Could you check a few things on this model? Use its own coordinates, in mm. A direction names the side the tool comes from. Coordinates: 2 decimals unless noted, no trailing zeros. Write each loop counter-clockwise with the first axis right and the second up, starting at its lowest first coordinate (ties: lowest second). Pieces come first, ordered by that corner, then holes.
Item 1: I want a section at B-B on z = 1.55. Please give me the cut outline in (x, y) (3 decimals).
Item 2: If I drill on probe 1 along Y at (x, z) = (9, 2.1) (3 decimals); probe 2 along X at (y, z) = (6.75, 0.6); probe 3 along X at (y, z) = (7.75, 0.65), over which ranges is the centre line in solid material (lowest first)?
Item 3: I want a section at A-A on x = 9.5. Please give me the cut outline in (y, z) (3 decimals), then the cut area to 3 significant figures.
Item 4: Thinking about a two-plate mould opening in X: for faces 3 (the flat face through (21, 6, 2.54)), 4 (the flat face through (34.29, 6, 1)), 5 (the cylindrical face through (3.176, 6.42, 1.288)), 6 (the flat face through (9, 3.175, 1)), which applies, +X half, -X half, draft (parallel to the pull), parting line (faces both ways), or undercut?
Item 5: I want a section at D-D on x = 27. Please give me the cut outline in (y, z), then the cut area to 3 significant figures.
Item 6: For P1, Ø1, axis at y = 4, z = 1, coming from the -X side, with a flat end and sliding along its axis, tell me the tip position at first contact or that it passes through.
Item 7: Which directions (+Z, -Z, +X, -X, +Y, -Y) give clear straight access to the entire face, cutting with the end or side of a thin tool? Please do faces 1 (the flat face through (21, 6, 0)), 2 (the cylindrical face through (15.874, 6.28, 1.288)).
Item 8: I want a section at C-C on y = 6. Please give me the cut outline in (x, z), then the cut area to 3 significant figures.
from build123d import *

# Parameters (mm, degrees)
F1_DEPTH = 2.54
F3_DEPTH = 2.541
F5_D     = 3.7973


with BuildPart() as f1:
    # F0 (on Top) → F1 (new body)
    with BuildSketch(Plane.XY):
        with BuildLine():
            ThreePointArc((0, 6.35), (1.8598719395, 1.8598719395), (6.35, 0))
            Line((6.35, 0), (34.29, 0))
            Line((34.29, 0), (34.29, 12.7))
            Line((34.29, 12.7), (6.35, 12.7))
            ThreePointArc((6.35, 12.7), (1.8598719395, 10.8401280605), (0, 6.35))
        make_face()
    extrude(amount=F1_DEPTH)

    # F2 (on face) → F3 (cut, through all)
    with BuildSketch(Plane.XY.offset(2.54)):
        with BuildLine():
            Line((12.7, 9.525), (6.35, 9.525))
            ThreePointArc((6.35, 9.525), (3.175, 6.35), (6.35, 3.175))
            Line((6.35, 3.175), (12.7, 3.175))
            ThreePointArc((12.7, 3.175), (15.875, 6.35), (12.7, 9.525))
        make_face()
    extrude(amount=-F3_DEPTH, mode=Mode.SUBTRACT)

    # F5 (through all)
    with Locations(Plane.XY.offset(2.54)):
        with Locations((27.305, 6.35)):
            Hole(F5_D / 2)


solid = f1.part
Response values:
1. outline: (6.35, 0) - (34.29, 0) - (34.29, 12.7) - (6.35, 12.7) arc R6.35 ccw to start; hole (6.35, 3.175) - (12.7, 3.175) arc R3.175 ccw to (12.7, 9.525) - (6.35, 9.525) arc R3.175 ccw to start; hole circle Ø3.797 at (27.305, 6.35)
2. probe 1: y = 0 to 3.175, 9.525 to 12.7
2. probe 2: x = 0.01 to 3.2, 15.85 to 25.45, 29.16 to 34.29
2. probe 3: x = 0.16 to 3.5, 15.55 to 26.02, 28.59 to 34.29
3. outline: (0, 0) - (3.175, 0) - (3.175, 2.54) - (0, 2.54) - close; (9.525, 0) - (12.7, 0) - (12.7, 2.54) - (9.525, 2.54) - close
3. area: 16.1 mm2
4. face 3: draft
4. face 4: +X half
4. face 5: undercut
4. face 6: undercut
5. outline: (0, 0) - (4.48, 0) - (4.48, 2.54) - (0, 2.54) - close; (8.22, 0) - (12.7, 0) - (12.7, 2.54) - (8.22, 2.54) - close
5. area: 22.7 mm2
6. P1: stops at x = 0.28
7. face 1: -Z, +X, -X, +Y, -Y
7. face 2: +Z, -Z
8. outline: (0.01, 0) - (3.19, 0) - (3.19, 2.54) - (0.01, 2.54) - close; (15.86, 0) - (25.44, 0) - (25.44, 2.54) - (15.86, 2.54) - close; (29.17, 0) - (34.29, 0) - (34.29, 2.54) - (29.17, 2.54) - close
8. area: 45.4 mm2
